The listing builds one solid part. Answer for the finished solid, in the listing's coordinates (mm). A direction names the side the tool comes from. Give positions to 0.01 mm unless a question says otherwise; leave off trailing zeros. Order: outer loops, then holes, each group sorted by start corner. A loop starts at its lowest first (then second) coordinate and runs counter-clockwise, first axis right, second up.
```python
from build123d import *

# Parameters (mm, degrees)
SKETCH1_W           = 107
SKETCH1_H           = 87.7
BOSS_EXTRUDE1_DEPTH = 13.85
SKETCH2_W           = 102.38
SKETCH2_H           = 83.08
CUT_EXTRUDE1_DEPTH  = 7.9
SKETCH4_R           = 2.5
SKETCH4_R_2         = 1.2
BOSS_EXTRUDE2_DEPTH = 6.2
SKETCH7_W           = 11.25
SKETCH7_H           = 4.8
BOSS_EXTRUDE3_DEPTH = 1.7
BOSS_EXTRUDE4_DEPTH = 3.15
CUT_EXTRUDE8_START  = -12
CUT_EXTRUDE8_DEPTH  = 20
BOSS_EXTRUDE7_DEPTH = 6
SKETCH24_W          = 8.731680323
SKETCH24_H          = 3
CUT_EXTRUDE10_DEPTH = 91.556729163
CHAMFER1_SIZE       = 1.5
CHAMFER2_SIZE       = 1.5


with BuildPart() as part:
    # Sketch1 → Boss-Extrude1 (new body)
    with BuildSketch(Plane(origin=(0, 0, 0), x_dir=(1, 0, 0), z_dir=(0, 1, 0))):
        Rectangle(SKETCH1_W, SKETCH1_H)
    extrude(amount=BOSS_EXTRUDE1_DEPTH)

    # Sketch2 → Cut-Extrude1 (cut)
    with BuildSketch(Plane(origin=(0, 13.85, 0), x_dir=(1, 0, 0), z_dir=(0, 1, 0))):
        Rectangle(SKETCH2_W, SKETCH2_H)
    extrude(amount=-CUT_EXTRUDE1_DEPTH, mode=Mode.SUBTRACT)

    # Sketch4 → Boss-Extrude2 (add)
    with BuildSketch(Plane(origin=(0, 5.95, 0), x_dir=(1, 0, 0), z_dir=(0, 1, 0))):
        with Locations((-42.5, -25)):
            Circle(SKETCH4_R)
        with Locations((-42.5, -25)):
            Circle(SKETCH4_R_2, mode=Mode.SUBTRACT)
        with Locations((42.5, 25)):
            Circle(SKETCH4_R)
        with Locations((42.5, 25)):
            Circle(SKETCH4_R_2, mode=Mode.SUBTRACT)
    extrude(amount=BOSS_EXTRUDE2_DEPTH)

    # Sketch7 → Boss-Extrude3 (add)
    with BuildSketch(Plane(origin=(-51.19, 0, 0), x_dir=(0, 0, -1), z_dir=(1, 0, 0))):
        with Locations((0, 8.35)):
            Rectangle(SKETCH7_W, SKETCH7_H)
    boss_extrude3 = extrude(amount=BOSS_EXTRUDE3_DEPTH)

    # Sketch8 → Boss-Extrude4 (add, symmetric)
    with BuildSketch(Plane.XY):
        Polygon((-49.49, 10.75), (-49.49, 18.75), (-50.99, 18.75), (-51.99, 16.75), (-51.19, 16.75), (-51.19, 10.75), align=None)
    boss_extrude4 = extrude(amount=BOSS_EXTRUDE4_DEPTH, both=True)

    # Mirror1: Boss-Extrude4 across plane
    add(boss_extrude4.mirror(Plane(origin=(0, 0, 0), x_dir=(0, 0, 1), z_dir=(1, 0, 0))))

    # Mirror2: Boss-Extrude3 across plane
    add(boss_extrude3.mirror(Plane(origin=(0, 0, 0), x_dir=(0, 0, 1), z_dir=(1, 0, 0))))

    # Sketch22 → Cut-Extrude8 (cut)
    with BuildSketch(Plane(origin=(0, 5.95, 0), x_dir=(1, 0, 0), z_dir=(0, 1, 0)).offset(CUT_EXTRUDE8_START)):
        Polygon((-51.19, 0), (-51.19, -6), (-53.5, -6), (-53.5, 6), (-51.19, 6), align=None)
    cut_extrude8 = extrude(amount=CUT_EXTRUDE8_DEPTH, mode=Mode.SUBTRACT)

    # Mirror3: Cut-Extrude8 across plane
    add(cut_extrude8.mirror(Plane(origin=(0, 0, 0), x_dir=(0, 0, 1), z_dir=(1, 0, 0))), mode=Mode.SUBTRACT)

    # Sketch23 → Boss-Extrude7 (add)
    with BuildSketch(Plane(origin=(0, 0, 0), x_dir=(-1, 0, 0), z_dir=(0, -1, 0))):
        Polygon((53.5, -43.85), (-53.5, -43.85), (-53.5, -14.731680323), (-37.056729163, -14.731680323), (-37.056729163, -6), (37.056729163, -6), (37.056729163, -14.731680323), (53.5, -14.731680323), align=None)
    boss_extrude7 = extrude(amount=BOSS_EXTRUDE7_DEPTH)

    # Sketch24 → Cut-Extrude10 (cut, through all)
    with BuildSketch(Plane(origin=(37.056729163, 0, 0), x_dir=(0, 0, -1), z_dir=(1, 0, 0))):
        with Locations((-10.365840161, -1.5)):
            Rectangle(SKETCH24_W, SKETCH24_H)
    cut_extrude10 = extrude(amount=-CUT_EXTRUDE10_DEPTH, mode=Mode.SUBTRACT)

    # Chamfer1
    chamfer1_edges = [part.edges().sort_by_distance(p)[0] for p in [
        (0, -3, 6),
    ]]
    chamfer(chamfer1_edges, length=CHAMFER1_SIZE)

    # Mirror4: Boss-Extrude7 across plane
    add(boss_extrude7.mirror(Plane.XY))

    # Mirror7: Cut-Extrude10 across plane
    add(cut_extrude10.mirror(Plane.XY), mode=Mode.SUBTRACT)

    # Chamfer2
    chamfer2_edges = [part.edges().sort_by_distance(p)[0] for p in [
        (0, -3, -6),
    ]]
    chamfer(chamfer2_edges, length=CHAMFER2_SIZE)


solid = part.part
```
1) Find section D-D (z = -25). Write down the section's boundary in (x, y), then the cut area to 3 significant figures.
Geometry says:
outline: (-53.5, -6) - (53.5, -6) - (53.5, 13.85) - (51.19, 13.85) - (51.19, 5.95) - (45, 5.95) - (45, 12.15) - (43.7, 12.15) - (43.7, 5.95) - (41.3, 5.95) - (41.3, 12.15) - (40, 12.15) - (40, 5.95) - (-51.19, 5.95) - (-51.19, 13.85) - (-53.5, 13.85) - close
area: 1,330 mm2
2) A tool of negligible diameter and unlimited length cuts with its end or side. For faces 5 (the cylindrical face through (43.61, 9.01, -24.54)), 6 (the flat face through (52, 7, -6)), 7 (the flat face through (50, 15, -3.15)), from which of +Z, -Z, +X, -X, +Y, -Y can it reach the whole face along a straight path? Write none if from no direction.
Geometry says:
face 5: +Y
face 6: +X, +Y, -Y
face 7: +X, -X, +Y
3) Find section B-B (z = -1.5). Write down the section's boundary in (x, y), then the cut area to 3 significant figures.
Geometry says:
outline: (-51.99, 16.75) - (-51.19, 16.75) - (-51.19, 0) - (51.19, 0) - (51.19, 16.75) - (51.99, 16.75) - (50.99, 18.75) - (49.49, 18.75) - (49.49, 5.95) - (-49.49, 5.95) - (-49.49, 18.75) - (-50.99, 18.75) - close
area: 654 mm2
4) Straight lines are drawn through the part: probe 1 along Z at (x, y) = (42.5, 9); probe 2 along X at (y, z) = (10.5, 25); probe 3 along X at (y, z) = (7.75, -25). For each, find the intervals that lie inside material, in ascending order.
Geometry says:
probe 1: z = -43.85 to -41.54, -27.5 to -26.2, -23.8 to -22.5, 41.54 to 43.85
probe 2: x = -53.5 to -51.19, -45 to -43.7, -41.3 to -40, 51.19 to 53.5
probe 3: x = -53.5 to -51.19, 40 to 41.3, 43.7 to 45, 51.19 to 53.5
5) Given P1, Ø9.5, axis at y = 8.5, z = -0.5, coming from the -X side; P2, Ø10, axis at x = 26, z = -25, coming from the +Y side; P3, Ø5, axis at y = 16, z = -15, coming from the -X side; P4, Ø0.9, axis at y = -4, z = 9.5, coming from the +X side, each flat-ended and moving along its own axis, determine where each tip first touches the part or whether it passes through.
Geometry says:
P1: stops at x = -51.19
P2: stops at y = 5.95
P3: stops at x = -53.5
P4: stops at x = 37.06
6) Find section C-C (x = 30). Write down the section's boundary in (y, z), then the cut area to 3 significant figures.
Geometry says:
outline: (-6, -43.85) - (13.85, -43.85) - (13.85, -41.54) - (5.95, -41.54) - (5.95, 41.54) - (13.85, 41.54) - (13.85, 43.85) - (-6, 43.85) - (-6, 6) - (-4.5, 6) - (-3, 7.5) - (-3, 14.73) - (0, 14.73) - (0, -14.73) - (-3, -14.73) - (-3, -7.5) - (-4.5, -6) - (-6, -6) - close
area: 958 mm2
7) Find section A-A (x = -38.5). Write down the section's boundary in (y, z), then the cut area to 3 significant figures.
Geometry says:
outline: (-6, -43.85) - (13.85, -43.85) - (13.85, -41.54) - (5.95, -41.54) - (5.95, 41.54) - (13.85, 41.54) - (13.85, 43.85) - (-6, 43.85) - (-6, 14.73) - (0, 14.73) - (0, -14.73) - (-6, -14.73) - close
area: 908 mm2
8) For a pull along Y with two mould halves and no side action, classify faces 1 (the flat face through (1, -2, -14.732)), 2 (the flat face through (-4, 13.85, -42)), 3 (the flat face through (-51.19, 10, -24)), 4 (the flat face through (1, -3, 11)) as +Y half, -Y half, draft (parallel to the pull), parting line (faces both ways), or undercut.
Geometry says:
face 1: undercut
face 2: +Y half
face 3: draft
face 4: undercut
